Read the model definition and answer for the solid it produces. Units are mm, in the model's axes. A direction names the side the tool comes from. Coordinates: 2 decimals unless noted, no trailing zeros. Use a Markdown table: item, result. Add a question column.
from build123d import *

# Parameters (mm, degrees)
CUT_EXTRUDE1_DEPTH      = 24.938835821
CUT_EXTRUDE1_DEPTH_BACK = 24.938835821
SKETCH2_W               = 8
SKETCH2_H               = 13
SKETCH2_H_2             = 10
CUT_EXTRUDE2_DEPTH      = 24.938835821
CUT_EXTRUDE2_DEPTH_BACK = 24.938835821
SKETCH3_R               = 1.5
CUT_EXTRUDE3_DEPTH      = 31.03444459
CUT_EXTRUDE4_START      = 10
CUT_EXTRUDE4_DEPTH      = 20


with BuildPart() as part:
    # Sketch1 → Revolve1 (revolve)
    with BuildSketch(Plane(origin=(0, 0, 0), x_dir=(0, 0, -1), z_dir=(1, 0, 0))):
        with BuildLine():
            Line((0, 20), (0, -20))
            Line((0, -20), (8, -20))
            add(Edge.make_bspline(
                [(8, 20), (10.604722665, 5.227883705), (8, -20)],
                knots=[0, 0, 0, 1, 1, 1], degree=2))
            Line((8, 20), (0, 20))
        make_face()
    revolve(axis=Axis((0, 20, 0), (0, -1, 0)))

    # Sketch2 → Cut-Extrude1 (cut, two sides: drawn at the far end of the back side and taken through both)
    with BuildSketch(Plane(origin=(0, 0, 0), x_dir=(0, 0, -1), z_dir=(1, 0, 0)).offset(-CUT_EXTRUDE1_DEPTH_BACK)):
        with Locations((0, 13.5)):
            Rectangle(SKETCH2_W, SKETCH2_H)
        with Locations((0, -15)):
            Rectangle(SKETCH2_W, SKETCH2_H_2)
    extrude(amount=CUT_EXTRUDE1_DEPTH + CUT_EXTRUDE1_DEPTH_BACK, mode=Mode.SUBTRACT)

    # Sketch3 → Cut-Extrude2 (cut, two sides: drawn at the far end of the back side and taken through both)
    with BuildSketch(Plane.XY.offset(-CUT_EXTRUDE2_DEPTH_BACK)):
        with Locations(Location((0, 15, 0), (0, 0, 270))):
            Circle(SKETCH3_R)
        with Locations(Location((0, -15, 0), (0, 0, 270))):
            Circle(SKETCH3_R)
    extrude(amount=CUT_EXTRUDE2_DEPTH + CUT_EXTRUDE2_DEPTH_BACK, mode=Mode.SUBTRACT)

    # Sketch4 → Cut-Extrude3 (cut, through all)
    with BuildSketch(Plane(origin=(0, 7, 0), x_dir=(1, 0, 0), z_dir=(0, 1, 0))):
        with BuildLine():
            ThreePointArc((-6.953963186, -2), (-6.568413105, -3.035383546), (-6.029726693, -4))
            Line((-6.029726693, -4), (6.029726693, -4))
            ThreePointArc((6.029726693, -4), (6.568413105, -3.035383546), (6.953963186, -2))
            ThreePointArc((6.953963186, -2), (7.165035811, -1.009884058), (7.235855443, 0))
            ThreePointArc((7.235855443, 0), (7.165035811, 1.009884058), (6.953963186, 2))
            ThreePointArc((6.953963186, 2), (6.568413105, 3.035383546), (6.029726693, 4))
            Line((6.029726693, 4), (-6.029726693, 4))
            ThreePointArc((-6.029726693, 4), (-6.568413105, 3.035383546), (-6.953963186, 2))
            ThreePointArc((-6.953963186, 2), (-7.235855443, 0), (-6.953963186, -2))
        make_face()
    extrude(amount=-CUT_EXTRUDE3_DEPTH, mode=Mode.SUBTRACT)

    # Sketch5 → Cut-Extrude4 (cut)
    with BuildSketch(Plane.XY.offset(CUT_EXTRUDE4_START)):
        with BuildLine():
            add(Edge.make_bspline(
                [(7.646286491, 15.644106168), (7.456972641, 17.101447086), (7.222625963, 18.553950368), (6.92820323, 20)],
                knots=[0.662887704, 0.662887704, 0.662887704, 0.662887704, 1, 1, 1, 1], degree=3))
            Line((6.92820323, 20), (2.687947329, 20))
            ThreePointArc((2.687947329, 20), (5.987907114, 18.756363324), (7.646286491, 15.644106168))
        make_face()
        with BuildLine():
            ThreePointArc((-7.646286491, 15.644106168), (-5.987907114, 18.756363324), (-2.687947329, 20))
            Line((-2.687947329, 20), (-6.92820323, 20))
            add(Edge.make_bspline(
                [(-6.92820323, 20), (-7.222625963, 18.553950368), (-7.456972641, 17.101447086), (-7.646286491, 15.644106168)],
                knots=[0, 0, 0, 0, 0.337112296, 0.337112296, 0.337112296, 0.337112296], degree=3))
        make_face()
    extrude(amount=-CUT_EXTRUDE4_DEPTH, mode=Mode.SUBTRACT)


solid = part.part
Item 1: Each of these flat-tipped pins is pushed along its axis until it touches: pin 1 (6 mm diameter, centred on x = -6.5, y = 4.5, fed in from -Z); pin 2 (6 mm diameter, centred on x = 4.5, z = 3, fed in from -Y); pin 3 (0.8 mm diameter, centred on x = 7, z = -0.5, fed in from -Y); pin 4 (8 mm diameter, centred on x = -5, y = -10, fed in from -Z). Where does it stop, or does it pass through?
Item 2: For faces 4 (the flat face through (-8, 7, 0)), 5 (the cylindrical face through (-4.664, 19.593, -5.35)), 6 (the flat face through (8, -10, 0)), determine the directions among +Z, -Z, +X, -X, +Y, -Y from which every point of the face is accessible in a straight line to the end or side of a thin tool.
Item 3: Consider probe 1 along Y at (x, z) = (0, -5.4); probe 2 along Z at (x, y) = (0.75, -9.5); probe 3 along Z at (x, y) = (-0.75, -1.5). Determine where each line is inside the solid, lowest interval first.
Item 4: Determine the mould class of faces 1 (the flat face through (-8, -10, 0)), 2 (the cylindrical face through (4.572, 19.631, 5.399)), 3 (the flat face through (0, 0, -4)) for opening direction X: pulls with the +X half, pulls with the -X half, needs draft (parallel to the pull), parting line crosses it, or undercut.
Item 5: Find section A-A on x = 0. Count the separate pieces of the cut face and the enclosed holes in it, then the cut area to 3 significant figures.
Geometry says:
| question | item | result |
|---|---|---|
| 1 | pin 1 | stops at z = -8.61 |
| 1 | pin 2 | stops at y = -20 |
| 1 | pin 3 | stops at y = -10 |
| 1 | pin 4 | stops at z = -8.86 |
| 2 | face 4 | +X, -X, +Y |
| 2 | face 5 | +Z, -Z, -X, +Y |
| 2 | face 6 | +X, -X, -Y |
| 3 | probe 1 | y = -20 to -16.5, -13.5 to 13.5, 16.5 to 20 |
| 3 | probe 2 | z = -8.86 to -4, 4 to 8.86 |
| 3 | probe 3 | z = -9.22 to -4, 4 to 9.22 |
| 4 | face 1 | needs draft |
| 4 | face 2 | pulls with the +X half |
| 4 | face 3 | undercut |
| 5 | separate pieces | 6 |
| 5 | enclosed holes | 0 |
| 5 | area | 334 mm2 |
